Drawing for the job (mm, zero at the part's lowest x, y, z). A direction names the side the tool comes from. Coordinates: 2 decimals unless noted, no trailing zeros. Order: outer loops, then holes, each group sorted by start corner. A loop starts at its lowest first (then second) coordinate and runs counter-clockwise, first axis right, second up. Notation, with made-up numbers: (79.25, -26) -> (102.25, -26) arc R14 ccw to (102.25, -3) -> close; hole circle Ø1 at (5, 53.5). An arc over 180 degrees is marked (long way). Write each question's results on one line, items separated by ' | '.
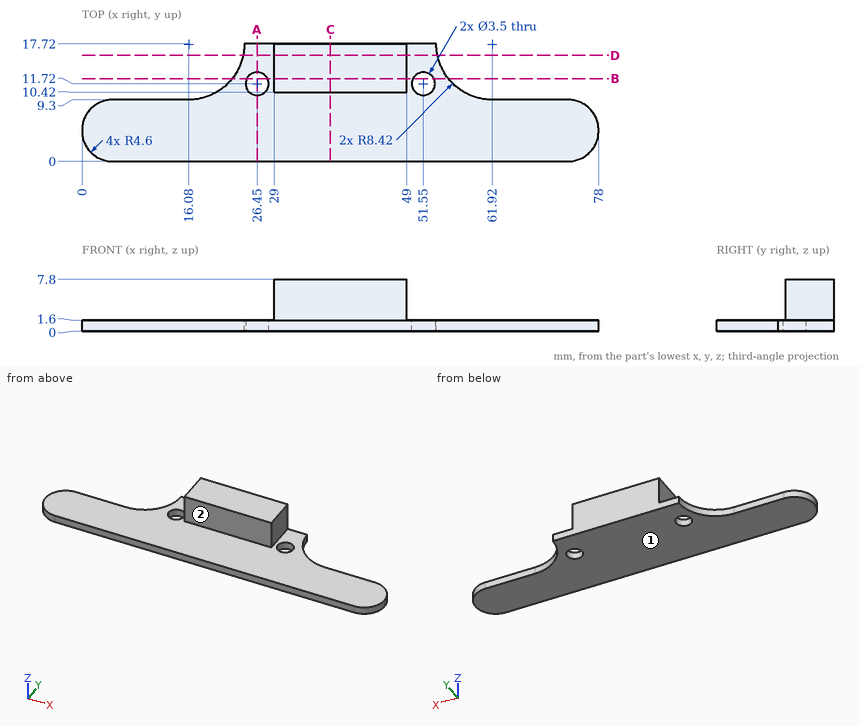
Item 1: Tool access for the marked faces 1 and 2: list every direction of +Z, -Z, +X, -X, +Y, -Y with a clear straight run to the whole face (end or side of a thin tool).
Answer:
face 1: -Z, +X, -X, +Y, -Y | face 2: +Z, +X, -X, -Y
Item 2: Drill centre lines: line 1 (Y direction, x = 51.55, z = 1.05); line 2 (X direction, y = 17, z = 5.75); line 3 (Z direction, x = 30, y = 3.5). Where is each one in solid material? Low to high. Write a range as from..to.
Answer:
line 1: y = 0..9.97, 13.47..17.72 | line 2: x = 29..49 | line 3: z = 0..1.6
Item 3: Pin check, flat tips, straight feed: pin 1 (6 mm diameter, centred on x = 60, y = 11.5, fed in from +Z); pin 2 (0.8 mm diameter, centred on x = 65.5, z = 1, fed in from +Y); pin 3 (3 mm diameter, centred on y = 15, z = 3.5, fed in from -X). Stop position of each tip, or through.
Answer:
pin 1: stops at z = 1.6 | pin 2: stops at y = 9.3 | pin 3: stops at x = 29
Item 4: Slice it at D-D, the plane y = 16. List the corners of the cut face in (x, z).
Answer:
outline: (24.32, 0) -> (53.68, 0) -> (53.68, 1.6) -> (49, 1.6) -> (49, 7.8) -> (29, 7.8) -> (29, 1.6) -> (24.32, 1.6) -> close
Item 5: Slice it at B-B, the plane y = 12.5. List the corners of the cut face in (x, z), and give its area (3 significant figures).
Answer:
outline: (22.69, 0) -> (24.88, 0) -> (24.88, 1.6) -> (22.69, 1.6) -> close; (28.02, 0) -> (49.98, 0) -> (49.98, 1.6) -> (49, 1.6) -> (49, 7.8) -> (29, 7.8) -> (29, 1.6) -> (28.02, 1.6) -> close; (53.12, 0) -> (55.31, 0) -> (55.31, 1.6) -> (53.12, 1.6) -> close | area: 166 mm^2
Item 6: Slice it at C-C, the plane x = 37.5. List the corners of the cut face in (y, z), and give its area (3 significant figures).
Answer:
outline: (0, 0) -> (17.72, 0) -> (17.72, 7.8) -> (10.42, 7.8) -> (10.42, 1.6) -> (0, 1.6) -> close | area: 73.6 mm^2
Item 7: Slice it at A-A, the plane x = 26.45. List the corners of the cut face in (y, z), and give its area (3 significant figures).
Answer:
outline: (0, 0) -> (9.97, 0) -> (9.97, 1.6) -> (0, 1.6) -> close; (13.47, 0) -> (17.72, 0) -> (17.72, 1.6) -> (13.47, 1.6) -> close | area: 22.8 mm^2
